```python
from build123d import *

# Parameters (mm, degrees)
SKETCH1_R                    = 19
SKETCH1_R_2                  = 1.5
SKETCH1_R_3                  = 8.5
BOSS_EXTRUDE1_DEPTH          = 12
BOSS_EXTRUDE2_DEPTH          = 4
BOSS_EXTRUDE2_DEPTH_BACK     = 12
SKETCH2_R                    = 21
SKETCH2_R_2                  = 19
BOSS_EXTRUDE3_START          = -5
SKETCH3_R                    = 3
SKETCH3_R_2                  = 1.5
BOSS_EXTRUDE3_DEPTH          = 5
CHAMFER1_SIZE                = 1
CIRPATTERN2_COUNT            = 4
CHAMFER1_OF_CIRPATTERN2_SIZE = 1
CHAMFER3_SIZE                = 1
SKETCH4_R                    = 2.5
CUT_EXTRUDE1_DEPTH           = 3


with BuildPart() as part:
    # Sketch1 → Boss-Extrude1 (new body)
    with BuildSketch(Plane(origin=(0, 0, 0), x_dir=(1, 0, 0), z_dir=(0, 1, 0))):
        with Locations(Location((0, 0, 0), (0, 0, 270))):
            Circle(SKETCH1_R)
        with Locations(Location((0, 15.5, 0), (0, 0, 270))):
            Circle(SKETCH1_R_2, mode=Mode.SUBTRACT)
        with Locations(Location((13.423393759, 7.75, 0), (0, 0, 270))):
            Circle(SKETCH1_R_2, mode=Mode.SUBTRACT)
        with Locations(Location((13.423393759, -7.75, 0), (0, 0, 270))):
            Circle(SKETCH1_R_2, mode=Mode.SUBTRACT)
        with Locations(Location((0, -15.5, 0), (0, 0, 270))):
            Circle(SKETCH1_R_2, mode=Mode.SUBTRACT)
        with Locations(Location((-13.423393759, -7.75, 0), (0, 0, 270))):
            Circle(SKETCH1_R_2, mode=Mode.SUBTRACT)
        with Locations(Location((-13.423393759, 7.75, 0), (0, 0, 270))):
            Circle(SKETCH1_R_2, mode=Mode.SUBTRACT)
        with Locations(Location((-2.75, 4.763139721, 0), (0, 0, 270))):
            Circle(SKETCH1_R_3, mode=Mode.SUBTRACT)
    extrude(amount=BOSS_EXTRUDE1_DEPTH)

    # Sketch2 → Boss-Extrude2 (add, two sides: drawn at the far end of the back side and taken through both)
    with BuildSketch(Plane.XZ.offset(-BOSS_EXTRUDE2_DEPTH_BACK)):
        with Locations(Location((0, 0, 0), (0, 0, 270))):
            Circle(SKETCH2_R)
        with Locations(Location((0, 0, 0), (0, 0, 270))):
            Circle(SKETCH2_R_2, mode=Mode.SUBTRACT)
    extrude(amount=BOSS_EXTRUDE2_DEPTH + BOSS_EXTRUDE2_DEPTH_BACK)

    # Sketch3 → Boss-Extrude3 (add)
    # profile 1 of 2: a face of its own
    with BuildSketch(Plane(origin=(0, 12, 0), x_dir=(1, 0, 0), z_dir=(0, 1, 0)).offset(BOSS_EXTRUDE3_START)):
        with Locations((0, 24.784609691)):
            Circle(SKETCH3_R)
        with Locations(Location((0, 24.784609691, 0), (0, 0, 270))):
            Circle(SKETCH3_R_2, mode=Mode.SUBTRACT)
    # profile 2 of 2: a face of its own
    with BuildSketch(Plane(origin=(0, 12, 0), x_dir=(1, 0, 0), z_dir=(0, 1, 0)).offset(BOSS_EXTRUDE3_START)):
        with BuildLine():
            ThreePointArc((3, 24.784609691), (0, 21.784609691), (-3, 24.784609691))
            Line((-3, 24.784609691), (-3, 20.784609691))
            ThreePointArc((-3, 20.784609691), (0, 21), (3, 20.784609691))
            Line((3, 20.784609691), (3, 24.784609691))
        make_face()
    boss_extrude3 = extrude(amount=BOSS_EXTRUDE3_DEPTH)

    # Chamfer1
    chamfer1_edges = [part.edges().sort_by_distance(p)[0] for p in [
        (0, 7, -26.284609691),
    ]]
    chamfer(chamfer1_edges, length=CHAMFER1_SIZE)

    # CirPattern2: Boss-Extrude3 ×4 about axis
    cirpattern2_axis = Axis((0, 0, 0), (0, 1, 0))
    for i in range(1, CIRPATTERN2_COUNT):
        add(boss_extrude3.rotate(cirpattern2_axis, i * 360 / CIRPATTERN2_COUNT))

    # Chamfer1 of CirPattern2
    chamfer1_of_cirpattern2_edges = [part.edges().sort_by_distance(p)[0] for p in [
        (-26.284609691, 7, 0),
        (0, 7, 26.284609691),
        (26.284609691, 7, 0),
    ]]
    chamfer(chamfer1_of_cirpattern2_edges, length=CHAMFER1_OF_CIRPATTERN2_SIZE)

    # Chamfer3
    chamfer3_edges = [part.edges().sort_by_distance(p)[0] for p in [
        (0, -4, 21),
        (-2.75, 0, -13.263139721),
        (-2.75, 12, -13.263139721),
    ]]
    chamfer(chamfer3_edges, length=CHAMFER3_SIZE)

    # Sketch4 → Cut-Extrude1 (cut)
    with BuildSketch(Plane(origin=(0, 12, 0), x_dir=(1, 0, 0), z_dir=(0, 1, 0))):
        with Locations(Location((-13.423393759, -7.75, 0), (0, 0, 270))):
            Circle(SKETCH4_R)
        with Locations(Location((-13.423393759, 7.75, 0), (0, 0, 270))):
            Circle(SKETCH4_R)
        with Locations(Location((0, 15.5, 0), (0, 0, 270))):
            Circle(SKETCH4_R)
        with Locations(Location((13.423393759, 7.75, 0), (0, 0, 270))):
            Circle(SKETCH4_R)
        with Locations(Location((13.423393759, -7.75, 0), (0, 0, 270))):
            Circle(SKETCH4_R)
        with Locations(Location((0, -15.5, 0), (0, 0, 270))):
            Circle(SKETCH4_R)
    extrude(amount=-CUT_EXTRUDE1_DEPTH, mode=Mode.SUBTRACT)


solid = part.part
```
Source: CAD feature listing. Evaluate the final solid. Frame: model axes, mm. A direction names the side the tool comes from. Give positions to 0.01 mm unless a question says otherwise; leave off trailing zeros. Loops run counter-clockwise (first coordinate to the right, second up) from the corner with the lowest first, then second, coordinate; pieces in that order, holes last. Notation, with made-up numbers: M 26.25,1.5 L 85.25,1.5 A23 ccw 85.25,14.5 Z; hole C -8,77 d4. An arc over 180 degrees is marked long. Put each result on its own line as item: value.
Q1. Pin query (flat end, axial travel): P1, Ø4, axis at x = 0.5, z = -16.5, coming from the +Y side; P2, Ø22, axis at x = -2.75, z = -4.76, coming from the -Y side; P3, Ø6, axis at y = 8.5, z = -11.5, coming from the +X side; P4, Ø6, axis at y = 0, z = 2, coming from the +X side. Return the tip coordinate at first contact, or that it passes through.
Response values:
P1: stops at y = 12
P2: stops at y = 0
P3: stops at x = 19.2
P4: stops at x = 21
Q2. Line query: probe 1 along X at (y, z) = (-0.9, 0); probe 2 along X at (y, z) = (2.25, 7.75); probe 3 along Z at (x, y) = (0, 1.25). Output: solid intervals per line, ascending. Write a range as [from, to].
Response values:
probe 1: x = [-21, -19], [19, 21]
probe 2: x = [-19.52, -14.92], [-11.92, 11.92], [14.92, 19.52]
probe 3: z = [-21, -17], [-14, -12.81], [3.28, 14], [17, 21]
Q3. Section A-A (y = 10.25). Count the separate pieces of the cut face and the enclosed holes in it, and give its area (3 significant figures).
Response values:
separate pieces: 1
enclosed holes: 11
area: 1,160 mm²
Q4. Reachability of faces 4 (the flat face through (-23, 9, -3)), 5 (the flat face through (-1, 9, 17)), 6 (the flat face through (3, 9, -23)) from +Z, -Z, +X, -X, +Y, -Y: full face, straight path, thin tool, end or side. Return the list, or none.
Response values:
face 4: -Z, -X, +Y, -Y
face 5: +Y
face 6: -Z, +X, +Y, -Y
Q5. Section C-C (y = 6.25). Return the cut outline in (x, z), and give its area (3 significant figures).
Response values:
outline: C 0,0 d42; hole C -13.42,-7.75 d3; hole C -13.42,7.75 d3; hole C -2.75,-4.76 d17; hole C 0,-15.5 d3; hole C 0,15.5 d3; hole C 13.42,-7.75 d3; hole C 13.42,7.75 d3
area: 1,120 mm²
Q6. Mould query, pull axis X, two halves, no side actions, for faces 1 (the cylindrical face through (-27.784, 9.465, -0.066)), 2 (the flat face through (4.25, 12, 1.93)), 3 (the cylindrical face through (11.96, 4.44, 7.42)). Classes: released by +X, released by -X, zero draft, split by the parting line, or undercut.
Response values:
face 1: released by -X
face 2: zero draft
face 3: undercut
